CAD build for the part. Positions are in the model's coordinates, mm. Face numbers are marked on the shaded views. Give positions to 0.01 mm unless a question says otherwise; leave off trailing zeros. Order: outer loops, then holes, each group sorted by start corner. A loop starts at its lowest first (then second) coordinate and runs counter-clockwise, first axis right, second up. Notation, with made-up numbers: (9, 58) -> (30, 58) arc R22 ccw to (30, 97) -> close; hole circle Ø11 at (1, -18). An arc over 180 degrees is marked (long way). Use one line per item in the form item = value. Start each with the question number.
1) Probe line 1 (X direction, y = 343, z = 0) (3 decimals); line 2 (Z direction, x = -18, y = 378.5); line 3 (X direction, y = 333, z = -37). List the from-to ranges inside material, lowest first.
2) Drop flat-ended pins along their axis: P1, Ø2, axis at y = 489.5, z = -7.5, coming from the +X side; P2, Ø1, axis at x = -38.5, y = 471.5, coming from the -Z side; P3, Ø8, axis at x = 44, y = 430, coming from the +Z side; P4, Ø2, axis at x = 0, y = 650.875, coming from the -Z side. Give the stop position or say it passes through.
3) Cut at A-A, the plane z = 0. Give the cut face in (x, y) (3 decimals).
4) Cut at C-C, the plane y = 571.5. Give the cut face in (x, z) (3 decimals), and give its area (3 significant figures).
5) Mould opens along Z. For the marked faces 1 and 2 say: pulls with the +Z half, pulls with the -Z half, needs draft (parallel to the pull), parting line crosses it, or undercut.
6) Cut at B-B, the plane x = 23. Give the cut face in (y, z).
from build123d import *

# Parameters (mm, degrees)
SKETCH1_R           = 63.5
SKETCH1_R_2         = 60.325
BOSS_EXTRUDE1_DEPTH = 660.4
SKETCH4_W           = 1.63195
SKETCH4_H           = 63.5
CIRPATTERN1_COUNT   = 6


with BuildPart() as part:
    # Sketch1 → Boss-Extrude1 (new body)
    with BuildSketch(Plane(origin=(0, 0, 0), x_dir=(1, 0, 0), z_dir=(0, 1, 0))):
        Circle(SKETCH1_R)
        Circle(SKETCH1_R_2, mode=Mode.SUBTRACT)
    extrude(amount=BOSS_EXTRUDE1_DEPTH)

    # Sketch4 → #4 Clearance Hole2 (revolve, cut)
    with BuildSketch(Plane(origin=(0, 650.875, 0), x_dir=(0, 1, 0), z_dir=(1, 0, 0))):
        with Locations((0.815975, 31.75)):
            Rectangle(SKETCH4_W, SKETCH4_H)
    f_4_clearance_hole2 = revolve(axis=Axis((0, 650.875, -6.35), (0, 0, 1)), mode=Mode.SUBTRACT)

    # CirPattern1: #4 Clearance Hole2 ×6 about axis
    cirpattern1_axis = Axis((0, 660.4, 0), (0, 1, 0))
    for i in range(1, CIRPATTERN1_COUNT):
        add(f_4_clearance_hole2.rotate(cirpattern1_axis, i * 360 / CIRPATTERN1_COUNT), mode=Mode.SUBTRACT)


solid = part.part
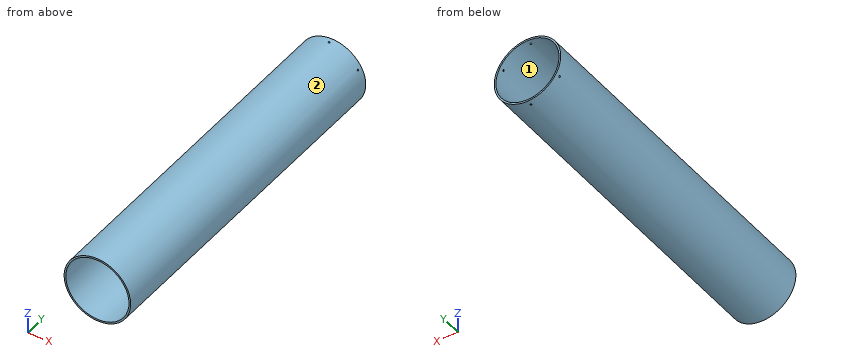
Result:
q1.line_1 = -63.5 to -60.325, 60.325 to 63.5
q1.line_2 = -60.9 to -57.58, 57.58 to 60.9
q1.line_3 = -51.61 to -47.65, 47.65 to 51.61
q2.P1 = 63.17
q2.P2 = -50.87
q2.P3 = 49.32
q2.P4 = through
q3.outline = (-63.5, 0) -> (-60.325, 0) -> (-60.325, 660.4) -> (-63.5, 660.4) -> close; (60.325, 0) -> (63.5, 0) -> (63.5, 660.4) -> (60.325, 660.4) -> close
q4.outline = circle Ø127 at (0, 0); hole circle Ø120.65 at (0, 0)
q4.area = 1,240 mm²
q5.face_1 = undercut
q5.face_2 = parting line crosses it
q6.outline = (0, -59.19) -> (660.4, -59.19) -> (660.4, -55.77) -> (0, -55.77) -> close; (0, 55.77) -> (660.4, 55.77) -> (660.4, 59.19) -> (0, 59.19) -> close
